Autodesk Inventor part; units mm, degrees
ref_plane "YZ Plane" through (0, 0, 0) normal (1, 0, 0) x (0, 1, 0)
ref_plane "XZ Plane" through (0, 0, 0) normal (0, 1, 0) x (-1, 0, 0)
ref_plane "XY Plane" through (0, 0, 0) normal (0, 0, 1) x (1, 0, 0)
sketch "Sketch1" plane through (0, 0, 0) normal (0, 1, 0) x (-1, 0, 0)
  line L0 (6.5, 4) -> (-6.5, 4)
  line L1 (-6.5, 4) -> (-6.5, -4)
  line L2 (-6.5, -4) -> (6.5, -4)
  line L3 (6.5, -4) -> (6.5, 4)
  line L4 (6.5, 4) -> (-6.5, -4) construction
  line L5 (-6.5, 4) -> (6.5, -4) construction
  point P0 (0, 0)
  dimension "d0" = 13
  dimension "d1" = 8
extrude "Extrusion1" add sketch "Sketch1" along normal blind 1
sketch "Sketch2" plane through (0, 1, 0) normal (0, 1, 0) x (1, 0, 0)
  line L0 (-6.5, 4) -> (-6.5, -4) construction
  line L1 (-6.5, 0) -> (-1.5, 0) construction
  circle A0 centre (-1.5, 0) radius 2.5
  point P0 (0, 0)
  dimension "d4" = 5
  dimension "d5" = 5
extrude "Extrusion2" cut sketch "Sketch2" against normal through all
properties part number "Rectangular Piece"
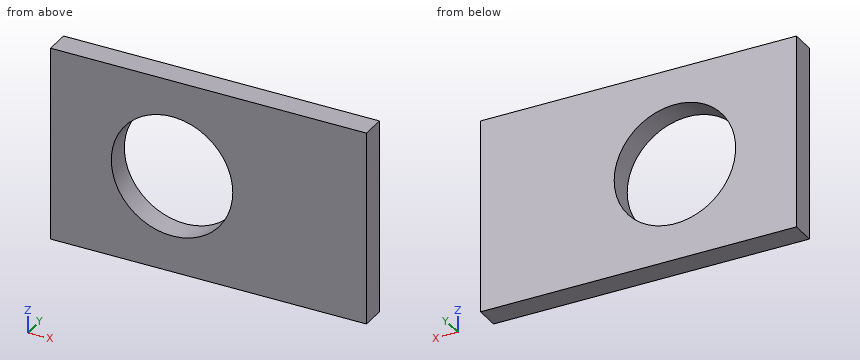
Check sheet for the modelled part. Datum: model origin and axes. Units: mm. Round coordinates to 2 decimals unless told otherwise and drop trailing zeros. Order: outer loops, then holes, each group sorted by start corner. A loop starts at its lowest first (then second) coordinate and runs counter-clockwise, first axis right, second up. Notation, with made-up numbers: (-7.5, 11.25) - (23.5, 11.25) arc R12 cw to (23.5, 17.25) - close; hole circle Ø6 at (33, 33.5). An arc over 180 degrees is marked (long way). Write item = value, one per line.
Q1. Section check B-B (z = 0). Record the boundary of the cut face in (x, y), and give its area (3 significant figures).
Computed:
outline = (-6.5, 0) - (-4, 0) - (-4, 1) - (-6.5, 1) - close; (1, 0) - (6.5, 0) - (6.5, 1) - (1, 1) - close
area = 8.00 mm^2
Q2. Thickness scan on line 1 along X through (y, z) = (0.65, 0); line 2 along Z through (x, y) = (-1.5, 0.7); line 3 along X through (y, z) = (0.4, -1.5). Record the ranges inside material, lowest first.
Computed:
line_1 = -6.5 to -4, 1 to 6.5
line_2 = -4 to -2.5, 2.5 to 4
line_3 = -6.5 to -3.5, 0.5 to 6.5
Q3. Section check C-C (y = 0.8). Record the boundary of the cut face in (x, z), and give its area (3 significant figures).
Computed:
outline = (-6.5, -4) - (6.5, -4) - (6.5, 4) - (-6.5, 4) - close; hole circle Ø5 at (-1.5, 0)
area = 84.4 mm^2
Q4. Section check A-A (x = -1.5). Record the boundary of the cut face in (y, z).
Computed:
outline = (0, -4) - (1, -4) - (1, -2.5) - (0, -2.5) - close; (0, 2.5) - (1, 2.5) - (1, 4) - (0, 4) - close
